Part model, mm, in its own coordinate system. Face numbers are marked on the shaded views. Round coordinates to 2 decimals unless told otherwise and drop trailing zeros. Write each loop counter-clockwise with the first axis right and the second up, starting at its lowest first coordinate (ties: lowest second). Pieces come first, ordered by that corner, then holes. Notation, with made-up numbers: M 18,9.25 L 51,9.25 A27 cw 51,43.25 Z; hole C -39,68 d5. An arc over 180 degrees is marked long. Use a Markdown table: item, result. Add a question column.
1) Slice it at A-A on y = 12.5. Write the cut outline in (x, z), plus the area to 3 significant figures.
2) Two-plate mould, pull along X, no slides. Class the marked faces 1, 2, 3 and 4: released by +X, released by -X, zero draft, split by the parting line, or undercut.
3) Slice it at B-B on x = 9.5. Write the cut outline in (y, z), plus the area to 3 significant figures.
4) Slice it at D-D on x = -1.75. Write the cut outline in (y, z), plus the area to 3 significant figures.
5) Drop a flat-ended pin along its axis: P1, Ø4.5, axis at y = 12.5, z = 0, coming from the +X side. Give the stop position or say it passes through.
6) Slice it at C-C on z = 5.25. Write the cut outline in (x, y), plus the area to 3 significant figures.
7) Wall check: probe 1 along Y at (x, z) = (0, -3.25); probe 2 along X at (y, z) = (12.5, 4.75); probe 3 along Z at (x, y) = (-2.5, 10.75). Give the ranges that are in metal, low to high.
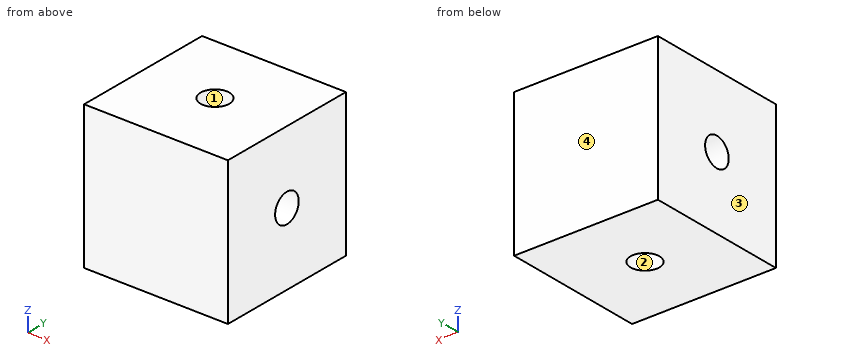
Autodesk Inventor part; units mm, degrees
ref_plane "YZ Plane" through (0, 0, 0) normal (1, 0, 0) x (0, 1, 0)
ref_plane "XZ Plane" through (0, 0, 0) normal (0, 1, 0) x (-1, 0, 0)
ref_plane "XY Plane" through (0, 0, 0) normal (0, 0, 1) x (1, 0, 0)
sketch "Sketch1" plane through (0, 0, 0) normal (0, 1, 0) x (-1, 0, 0)
  line L0 (12.5, -12.5) -> (-12.5, -12.5)
  line L1 (-12.5, -12.5) -> (-12.5, 12.5)
  line L2 (-12.5, 12.5) -> (12.5, 12.5)
  line L3 (12.5, 12.5) -> (12.5, -12.5)
  line L4 (12.5, -12.5) -> (-12.5, 12.5) construction
  line L5 (-12.5, -12.5) -> (12.5, 12.5) construction
  point P0 (0, 0)
  dimension "d0" = 25
  dimension "d1" = 25
extrude "Extrusion1" add sketch "Sketch1" along normal blind 25
sketch "Sketch2" plane through (12.5, 0, 12.5) normal (1, 0, 0) x (0, 0, -1)
  line L0 (0, 0) -> (25, 0)
  line L1 (0, 0) -> (25, 25)
  circle A0 centre (12.5, 12.5) radius 2.5
  point P0 (12.5, 0)
  dimension "d4" = 5
extrude "Extrusion2" cut sketch "Sketch2" against normal blind 25
sketch "Sketch3" plane through (-12.5, 0, 12.5) normal (0, 0, 1) x (1, 0, 0)
  line L0 (25, 25) -> (0, 25)
  line L1 (25, 0) -> (25, 25)
  line L2 (0, 25) -> (25, 0)
  circle A0 centre (12.5, 12.5) radius 2.5
  point P0 (12.5, 0)
  dimension "d7" = 5
extrude "Extrusion3" cut sketch "Sketch3" against normal blind 25 contours A0 L2 | L2 A0
properties part number "coupling"
Entries:
| question | item | result |
|---|---|---|
| 1 | outline | M -12.5,-12.5 L -2.5,-12.5 L -2.5,-2.5 L -12.5,-2.5 Z; M -12.5,2.5 L -2.5,2.5 L -2.5,12.5 L -12.5,12.5 Z; M 2.5,-12.5 L 12.5,-12.5 L 12.5,-2.5 L 2.5,-2.5 Z; M 2.5,2.5 L 12.5,2.5 L 12.5,12.5 L 2.5,12.5 Z |
| 1 | area | 400 mm^2 |
| 2 | face 1 | undercut |
| 2 | face 2 | undercut |
| 2 | face 3 | released by -X |
| 2 | face 4 | zero draft |
| 3 | outline | M 0,-12.5 L 25,-12.5 L 25,12.5 L 0,12.5 Z; hole C 12.5,0 d5 |
| 3 | area | 605 mm^2 |
| 4 | outline | M 0,-12.5 L 10.71,-12.5 L 10.71,-1.75 A2.5 cw 10.71,1.75 L 10.71,12.5 L 0,12.5 Z; M 14.29,-12.5 L 25,-12.5 L 25,12.5 L 14.29,12.5 L 14.29,1.75 A2.5 cw 14.29,-1.75 Z |
| 4 | area | 532 mm^2 |
| 5 | P1 | passes through |
| 6 | outline | M -12.5,0 L 12.5,0 L 12.5,25 L -12.5,25 Z; hole C 0,12.5 d5 |
| 6 | area | 605 mm^2 |
| 7 | probe 1 | y = 0 to 10, 15 to 25 |
| 7 | probe 2 | x = -12.5 to -2.5, 2.5 to 12.5 |
| 7 | probe 3 | z = -12.5 to -1.79, 1.79 to 12.5 |
